Part model, mm, in its own coordinate system. Give positions to 0.01 mm unless a question says otherwise; leave off trailing zeros. Write each loop counter-clockwise with the first axis right and the second up, starting at its lowest first coordinate (ties: lowest second). Pieces come first, ordered by that corner, then holes. Notation, with made-up numbers: (33, 75) - (64, 75) arc R11 cw to (64, 92) - close; hole circle Ø6 at (-35, 51). An arc over 180 degrees is marked (long way). Answer as a JSON object with one key per item and string values. Group by question number.
```python
from build123d import *

# Parameters (mm, degrees)
F1_DEPTH = 6.35
F2_D     = 12.7


# Not quite as in the source:
# - a feature names something its author has since deleted; it is built from what else it names


with BuildPart() as f1:
    # F0 (on Right) → F1 (new body)
    with BuildSketch(Plane.YZ):
        Polygon((-73.2459126534, -2.6395988316), (-73.2459126534, -45.580811482), (-22.4459126534, -74.9102051568), (-22.4459126534, 26.6897948432), align=None)
    extrude(amount=F1_DEPTH)

    # F2 (through all)
    with Locations(Plane(origin=(0, 0, 0), x_dir=(0, 1, 0), z_dir=(-1, 0, 0))):
        with Locations((-60.5459126534, 24.1152988316)):
            Hole(F2_D / 2)


solid = f1.part
```
1) Drill centre lines: line 1 along Z through (x, y) = (4.5, -59); line 2 along Z through (x, y) = (1.75, -57.5); line 3 along Y through (x, z) = (0.5, -19.5). Where is each one in solid material? Low to high. Write a range as from..to.
2) Two-plate mould, pull along Y, no slides. Class faces 1 (the flat face through (3.13, -47.49, 12.23)), 2 (the flat face through (3, -22.446, -25)), 3 (the cylindrical face through (3.22, -54.2, -24.39)): +Y half, -Y half, draft (parallel to the pull), parting line (faces both ways), or undercut.
3) Saw through at A-A (y = -58). List the corners of the cut face in (x, z).
4) Drop flat-ended pins along their axis: P1, Ø2, axis at x = 1, y = -42, coming from the -Z side; P2, Ø10, axis at y = -60.55, z = -24.12, coming from the +X side. Give the stop position or say it passes through.
5) Saw through at C-C (z = 0.5). List the corners of the cut face in (x, y), and give its area (3 significant figures).
6) Saw through at D-D (y = -37). List the corners of the cut face in (x, z), and give its area (3 significant figures).
7) Saw through at B-B (x = 4.75). List the corners of the cut face in (y, z).
Checks:
{
 "1": {"line 1": "-53.81..-30.27, -17.96..5.59", "line 2": "-54.67..-29.69, -18.54..6.45", "line 3": "-73.25..-64.91, -56.18..-22.45"},
 "2": {"face 1": "-Y half", "face 2": "+Y half", "face 3": "undercut"},
 "3": {"outline": "(0, -54.38) - (6.35, -54.38) - (6.35, -29.93) - (0, -29.93) - close; (0, -18.3) - (6.35, -18.3) - (6.35, 6.16) - (0, 6.16) - close"},
 "4": {"P1": "z = -64.2", "P2": "through"},
 "5": {"outline": "(0, -67.81) - (6.35, -67.81) - (6.35, -22.45) - (0, -22.45) - close", "area": "288 mm2"},
 "6": {"outline": "(0, -66.51) - (6.35, -66.51) - (6.35, 18.29) - (0, 18.29) - close", "area": "538 mm2"},
 "7": {"outline": "(-73.25, -45.58) - (-22.45, -74.91) - (-22.45, 26.69) - (-73.25, -2.64) - close; hole circle Ø12.7 at (-60.55, -24.12)"}
}
